Source: CAD feature listing. Evaluate the final solid. Frame: model axes, mm. A direction names the side the tool comes from. Round coordinates to 2 decimals unless told otherwise and drop trailing zeros. Order: outer loops, then holes, each group sorted by start corner. A loop starts at its lowest first (then second) coordinate and runs counter-clockwise, first axis right, second up. Notation, with made-up numbers: (2, 68) -> (9, 68) arc R22 ccw to (9, 105) -> close; hole circle Ø11 at (87.5, -30). An arc over 180 degrees is marked (long way). Write item = value, one per line. Start each with the question number.
(1) Cut plane A-A on z = -32.5. Return the cut outline in (x, y).
(2) Cut plane C-C on z = -47.5. Return the cut outline in (x, y), then the cut area to 3 significant figures.
(3) Cut plane B-B on x = -39. Return the cut outline in (y, z).
(4) Draft query along X for faces 1 (the face through (-49.94, 1.58, -22.26)), 2 (the face through (26.46, 1.58, -20.03)), 3 (the face through (-53.81, 1.58, -21.12)), 4 (the face through (-31.154, 2, -52)). Return one class per face: released by +X, released by -X, zero draft, split by the parting line, or undercut.
(5) Ray query, line 1 (Z direction, x = 20, y = 2); line 2 (Z direction, x = -53, y = 0.45); line 3 (X direction, y = 1.85, z = -32.5). Return the intervals inside material, ascending.
(6) Contact query for flat-ended pins moving along their axis: pin 1 Ø3 at (x, z) = (-14, -30.5) entering from -Y; pin 2 Ø1 at (y, z) = (1, -53) entering from +X; pin 3 Ø1.6 at (y, z) = (1.5, -51) entering from -X; pin 4 Ø1.6 at (x, y) = (-9.5, 1) entering from -Z. Output: stop coordinate, or through.
(7) Reachability of faces 5 (the face through (-45.49, 1.58, 24.26)), 6 (the face through (-38.48, 1.58, 31.67)), 7 (the face through (-44.39, 1.58, -33.36)) from +Z, -Z, +X, -X, +Y, -Y: full face, straight path, thin tool, end or side. Return the list, or none.
from build123d import *

# Parameters (mm, degrees)
BOSS_EXTRUDE1_DEPTH = 3.2


with BuildPart() as part:
    # Sketch1 → Boss-Extrude1 (new body)
    with BuildSketch(Plane(origin=(0, 0, 0), x_dir=(1, 0, 0), z_dir=(0, 1, 0))):
        Polygon((5.369694579, -35.29298371), (8.947903919, -28.137816492), (13.960969185, -31.527970224), (16.734685449, -25.98150779), (11.721620183, -22.591354059), (14.495336447, -17.044891626), (19.508401713, -20.435045357), (22.282117977, -14.888582924), (17.269052711, -11.498429192), (20.042768975, -5.951966759), (25.055834241, -9.34212049), (27.829550505, -3.795658057), (22.816485239, -0.405504326), (26.394694579, 6.749662892), (22.816485239, 13.90483011), (27.829550505, 17.294983841), (25.055834241, 22.841446275), (20.042768975, 19.451292543), (17.269052711, 24.997754977), (22.282117977, 28.387908708), (19.508401713, 33.934371141), (14.495336447, 30.54421741), (11.721620183, 36.090679843), (16.734685449, 39.480833575), (13.960969185, 45.027296008), (8.947903919, 41.637142277), (5.369694579, 48.792309495), (-0.14692929, 48.792309495), (-0.14692929, 54.792309495), (-6.348279742, 54.792309495), (-6.348279742, 48.792309495), (-12.549630195, 48.792309495), (-12.549630195, 54.792309495), (-18.750980648, 54.792309495), (-18.750980648, 48.792309495), (-24.9523311, 48.792309495), (-24.9523311, 54.792309495), (-31.153681553, 54.792309495), (-31.153681553, 48.792309495), (-36.670305421, 48.792309495), (-40.248514761, 41.637142277), (-45.261580028, 45.027296008), (-48.035296291, 39.480833575), (-43.022231025, 36.090679843), (-45.795947289, 30.54421741), (-50.809012555, 33.934371141), (-53.582728819, 28.387908708), (-48.569663553, 24.997754977), (-51.343379817, 19.451292543), (-56.356445083, 22.841446275), (-59.130161347, 17.294983841), (-54.117096081, 13.90483011), (-57.695305421, 6.749662892), (-54.117096081, -0.405504326), (-59.130161347, -3.795658057), (-56.356445083, -9.34212049), (-51.343379817, -5.951966759), (-48.569663553, -11.498429192), (-53.582728819, -14.888582924), (-50.809012555, -20.435045357), (-45.795947289, -17.044891626), (-43.022231025, -22.591354059), (-48.035296291, -25.98150779), (-45.261580028, -31.527970224), (-40.248514761, -28.137816492), (-36.670305421, -35.29298371), align=None)
    extrude(amount=BOSS_EXTRUDE1_DEPTH)


solid = part.part
Evaluation:
q1.outline = (-51.53, 0) -> (-48.69, 0) -> (-48.69, 3.2) -> (-51.53, 3.2) -> close; (-44.82, 0) -> (13.52, 0) -> (13.52, 3.2) -> (-44.82, 3.2) -> close; (17.39, 0) -> (20.23, 0) -> (20.23, 3.2) -> (17.39, 3.2) -> close
q2.outline = (-37.32, 0) -> (6.02, 0) -> (6.02, 3.2) -> (-37.32, 3.2) -> close
q2.area = 139 mm^2
q3.outline = (0, -44.13) -> (3.2, -44.13) -> (3.2, 30.63) -> (0, 30.63) -> close
q4.face_1 = undercut
q4.face_2 = released by +X
q4.face_3 = undercut
q4.face_4 = released by -X
q5.line_1 = -32.95 to -26.84, -19.54 to 6.04, 13.35 to 19.45
q5.line_2 = -29.55 to -27.99, -20.57 to 7.07, 14.49 to 16.05
q5.line_3 = -51.53 to -48.69, -44.82 to 13.52, 17.39 to 20.23
q6.pin_1 = 0
q6.pin_2 = -0.15
q6.pin_3 = -31.15
q6.pin_4 = -48.79
q7.face_5 = -X, +Y, -Y
q7.face_6 = +Z, +Y, -Y
q7.face_7 = +Y, -Y
